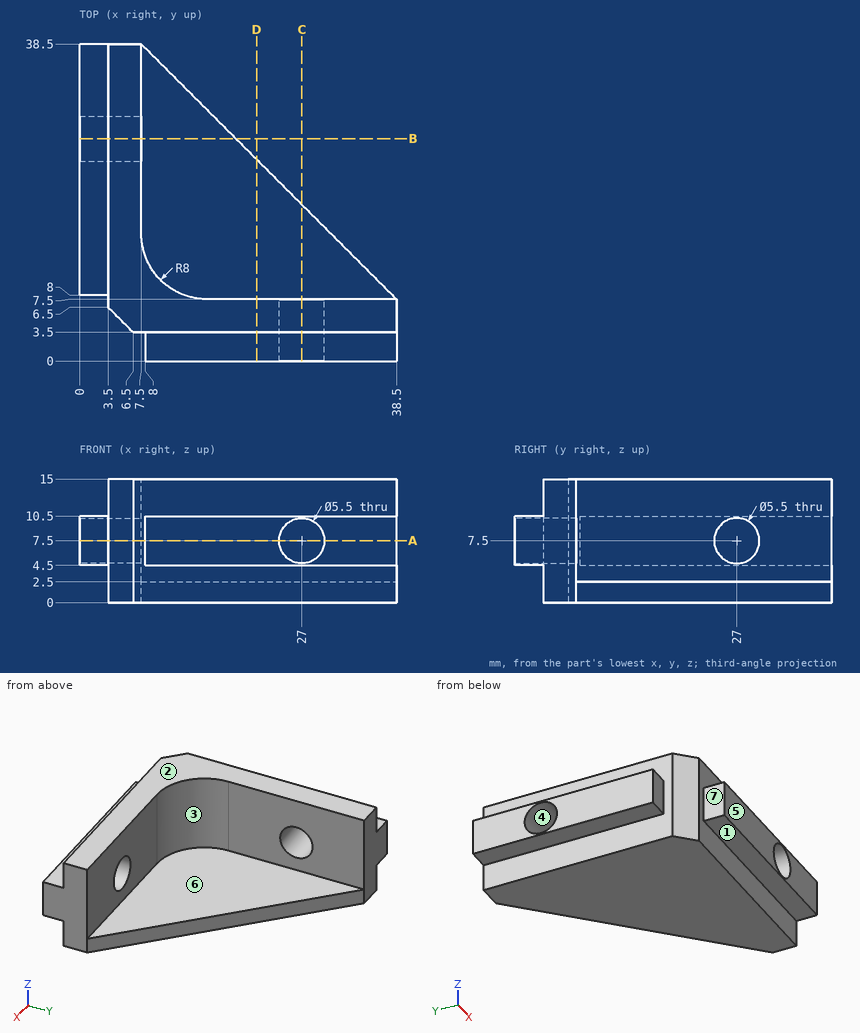
Here's the drawing with two shaded views (mm, measured from the low corner). I have some questions. A direction names the side the tool comes from. Round coordinates to 2 decimals unless told otherwise and drop trailing zeros. Loops run counter-clockwise (first coordinate to the right, second up) from the corner with the lowest first, then second, coordinate; pieces in that order, holes last.
1. Will these pins go through, and if not, where does the flat tip stop? pin 1 (9.5 mm diameter, centred on x = 16.5, y = 21.5, fed in from +Z); pin 2 (4 mm diameter, centred on x = 1, y = 21, fed in from -Z); pin 3 (1 mm diameter, centred on x = 2, y = 20, fed in from +Z); pin 4 (1.5 mm diameter, centred on x = 8, z = 4.5, fed in from -Y).
Answers:
pin 1: stops at z = 2.5
pin 2: stops at z = 4.5
pin 3: stops at z = 10.5
pin 4: stops at y = 0
2. Suppose I cut it at D-D, the plane x = 21.5. Please give me the cut outline in (y, z), and give its area (4 significant figures).
Answers:
outline: (0, 4.5) - (3.5, 4.5) - (3.5, 0) - (24.5, 0) - (24.5, 2.5) - (7.5, 2.5) - (7.5, 15) - (3.5, 15) - (3.5, 10.5) - (0, 10.5) - close
area: 123.5 mm2
3. Suppose I cut it at A-A, the plane z = 7.5. Please give me the cut outline in (x, y), and give its area (3 significant figures).
Answers:
outline: (0, 8) - (3.5, 8) - (3.5, 6.5) - (6.5, 3.5) - (8, 3.5) - (8, 0) - (24.25, 0) - (24.25, 7.5) - (15.5, 7.5) arc R8 cw to (7.5, 15.5) - (7.5, 24.25) - (0, 24.25) - close; (0, 29.75) - (7.5, 29.75) - (7.5, 38.5) - (0, 38.5) - close; (29.75, 0) - (38.5, 0) - (38.5, 7.5) - (29.75, 7.5) - close
area: 404 mm2
4. If I drill on probe 1 along Y at (x, z) = (2.5, 7.5); probe 2 along Z at (x, y) = (10.5, 15.5); probe 3 along X at (y, z) = (19.5, 14.25), over which ranges is the centre line in solid material (lowest first)?
Answers:
probe 1: y = 8 to 24.25, 29.75 to 38.5
probe 2: z = 0 to 2.5
probe 3: x = 3.5 to 7.5
5. Thinking about a two-plate mould opening in Z: for the marked faces 1, 2, 3 and 4, which applies, released by +Z, released by -Z, zero draft, split by the parting line, or undercut?
Answers:
face 1: released by -Z
face 2: released by +Z
face 3: zero draft
face 4: undercut
6. For the marked faces 5, 6 and 7, which set-ups out of +Z, -Z, +X, -X, +Y, -Y let a thin tool reach every point of the face, with its end or its side?
Answers:
face 5: +Z, -Z, +X, -X, -Y
face 6: +Z, +X, +Y
face 7: +Z, -Z, -X, -Y
7. Suppose I cut it at B-B, the plane y = 27. Please give me the cut outline in (x, z).
Answers:
outline: (0, 4.5) - (3.5, 4.5) - (3.5, 0) - (19, 0) - (19, 2.5) - (7.5, 2.5) - (7.5, 4.75) - (0, 4.75) - close; (0, 10.25) - (7.5, 10.25) - (7.5, 15) - (3.5, 15) - (3.5, 10.5) - (0, 10.5) - close
